Here's how the part is built. I have some questions about the finished solid (model axes, mm). Face numbers are marked on the shaded views. A direction names the side the tool comes from. Give positions to 0.01 mm unless a question says otherwise; leave off trailing zeros. Loops run counter-clockwise (first coordinate to the right, second up) from the corner with the lowest first, then second, coordinate; pieces in that order, holes last. Notation, with made-up numbers: (70, 82.5) -> (110, 82.5) arc R17 cw to (110, 105.5) -> close; hole circle Ø4 at (62, 48.25). An arc over 180 degrees is marked (long way). Answer in a Markdown table with one row per item. Add a question column.
Item 1: Which directions (+Z, -Z, +X, -X, +Y, -Y) give clear straight access to the entire face, cutting with the end or side of a thin tool? Please do the marked faces 1 and 2.
Item 2: For P1, Ø3, axis at x = 35.5, z = -2, coming from the +Y side; P2, Ø5, axis at y = -3.5, z = -0.5, coming from the -X side; P3, Ø4, axis at x = 37, y = -3.5, coming from the +Z side; P4, Ø3, axis at x = 26, z = 2.5, coming from the -Y side, each with a flat end and sliding along its axis, tell me the tip position at first contact or that it passes through.
Item 3: If we section it at A-A (y = 0): Write out the boundary of the cut face in (x, z) (3 decimals).
Item 4: If we section it at B-B (x = 11): Write out the boundary of the cut face in (y, z).
Item 5: If I drill on line 1 (X direction, y = -1, z = -0.75); line 2 (Y direction, x = 26, z = -2); line 3 (X direction, y = -3.5, z = -1), over which ranges is the centre line in solid material (lowest first)?
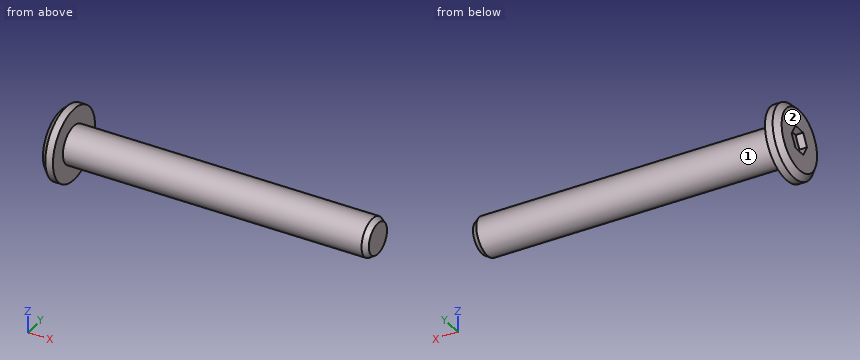
```python
from build123d import *

# Parameters (mm, degrees)
CUT_EXTRUDE1_DEPTH = 1
CHAMFER1_SIZE      = 0.75


with BuildPart() as part:
    # Sketch1 → Revolve1 (revolve)
    with BuildSketch(Plane.XY):
        Polygon((41.75, 0), (41.75, 2.057236169), (41.055, 2.5), (1.75, 2.5), (1.75, 4.75), (0, 4.75), (0, 0), align=None)
    revolve(axis=Axis((0, 0, 0), (1, 0, 0)))

    # Sketch5 → Cut-Extrude1 (cut)
    with BuildSketch(Plane.ZY):
        Polygon((1.5, -0.866025404), (1.5, 0.866025404), (0, 1.732050808), (-1.5, 0.866025404), (-1.5, -0.866025404), (0, -1.732050808), align=None)
    extrude(amount=-CUT_EXTRUDE1_DEPTH, mode=Mode.SUBTRACT)

    # Chamfer1
    chamfer1_edges = [part.edges().sort_by_distance(p)[0] for p in [
        (0, -4.75, 0),
    ]]
    chamfer(chamfer1_edges, length=CHAMFER1_SIZE)


solid = part.part
```
Recorded:
| question | item | result |
|---|---|---|
| 1 | face 1 | +X |
| 1 | face 2 | +Z, -Z, -X, +Y, -Y |
| 2 | P1 | stops at y = 2.45 |
| 2 | P2 | stops at x = 0 |
| 2 | P3 | stops at z = 2 |
| 2 | P4 | stops at y = -2.29 |
| 3 | outline | (0, -4) -> (0.75, -4.75) -> (1.75, -4.75) -> (1.75, -2.5) -> (41.055, -2.5) -> (41.75, -2.057) -> (41.75, 2.057) -> (41.055, 2.5) -> (1.75, 2.5) -> (1.75, 4.75) -> (0.75, 4.75) -> (0, 4) -> (0, 1.5) -> (1, 1.5) -> (1, -1.5) -> (0, -1.5) -> close |
| 4 | outline | circle Ø5 at (0, 0) |
| 5 | line 1 | x = 1 to 41.75 |
| 5 | line 2 | y = -1.5 to 1.5 |
| 5 | line 3 | x = 0 to 1.75 |
